Could you check a few things on this model? Use its own coordinates, in mm. A direction names the side the tool comes from. Coordinates: 2 decimals unless noted, no trailing zeros. Loops run counter-clockwise (first coordinate to the right, second up) from the corner with the lowest first, then second, coordinate; pieces in that order, holes last. Notation, with made-up numbers: (-15.5, -10.75) - (2.5, -10.75) arc R28 cw to (2.5, 23.25) - close; hole circle Ø2 at (10.5, 86.5). An arc over 180 degrees is marked (long way). Put each result on its own line as item: value. Start each with the question number.
```python
from build123d import *

# Parameters (mm, degrees)
SKETCH1_W           = 30
SKETCH1_H           = 30
SKETCH1_W_2         = 20
SKETCH1_H_2         = 20
BOSS_EXTRUDE1_DEPTH = 20
BOSS_EXTRUDE2_START = 20
SKETCH1_2_W         = 30
SKETCH1_2_H         = 30
SKETCH1_2_W_2       = 20
SKETCH1_2_H_2       = 20
BOSS_EXTRUDE2_DEPTH = 10
SKETCH3_R           = 2.5
CUT_EXTRUDE1_DEPTH  = 46
SKETCH3_3_R         = 4
SKETCH3_3_R_2       = 2.5
CUT_EXTRUDE2_DEPTH  = 3
CUT_EXTRUDE3_START  = -27
SKETCH3_4_R         = 4
SKETCH3_4_R_2       = 2.5
CUT_EXTRUDE3_DEPTH  = 3
SKETCH4_W           = 10
SKETCH4_H           = 30
BOSS_EXTRUDE3_DEPTH = 50
SKETCH5_R           = 2.5
CUT_EXTRUDE4_DEPTH  = 84.815273071
LPATTERN1_COUNT     = 6
LPATTERN1_PITCH     = 7.5
FILLET1_R           = 15


with BuildPart() as part:
    # Sketch1 → Boss-Extrude1 (new body)
    with BuildSketch(Plane(origin=(0, 0, 0), x_dir=(1, 0, 0), z_dir=(0, 1, 0))):
        Rectangle(SKETCH1_W, SKETCH1_H)
        Rectangle(SKETCH1_W_2, SKETCH1_H_2, mode=Mode.SUBTRACT)
    extrude(amount=BOSS_EXTRUDE1_DEPTH)

    # Sketch1<2> → Boss-Extrude2 (add)
    # profile 1 of 2: a face of its own
    with BuildSketch(Plane(origin=(0, 0, 0), x_dir=(1, 0, 0), z_dir=(0, 1, 0)).offset(BOSS_EXTRUDE2_START)):
        Rectangle(SKETCH1_2_W, SKETCH1_2_H)
        Rectangle(SKETCH1_2_W_2, SKETCH1_2_H_2, mode=Mode.SUBTRACT)
    # profile 2 of 2: a face of its own
    with BuildSketch(Plane(origin=(0, 0, 0), x_dir=(1, 0, 0), z_dir=(0, 1, 0)).offset(BOSS_EXTRUDE2_START)):
        Rectangle(SKETCH1_2_W_2, SKETCH1_2_H_2)
    extrude(amount=BOSS_EXTRUDE2_DEPTH)

    # Sketch3 → Cut-Extrude1 (cut, through all)
    with BuildSketch(Plane(origin=(15, 0, 0), x_dir=(0, 0, -1), z_dir=(1, 0, 0))):
        with Locations((0, 15)):
            Circle(SKETCH3_R)
    extrude(amount=-CUT_EXTRUDE1_DEPTH, mode=Mode.SUBTRACT)

    # Sketch3<3> → Cut-Extrude2 (cut)
    # profile 1 of 2: a face of its own
    with BuildSketch(Plane(origin=(15, 0, 0), x_dir=(0, 0, -1), z_dir=(1, 0, 0))):
        Polygon((-5, 17.886751346), (-5, 12.113248654), (0, 9.226497308), (5, 12.113248654), (5, 17.886751346), (0, 20.773502692), align=None)
        with Locations((0, 15)):
            Circle(SKETCH3_3_R, mode=Mode.SUBTRACT)
    # profile 2 of 2: a face of its own
    with BuildSketch(Plane(origin=(15, 0, 0), x_dir=(0, 0, -1), z_dir=(1, 0, 0))):
        with Locations((0, 15)):
            Circle(SKETCH3_3_R)
        with Locations((0, 15)):
            Circle(SKETCH3_3_R_2, mode=Mode.SUBTRACT)
    extrude(amount=-CUT_EXTRUDE2_DEPTH, mode=Mode.SUBTRACT)

    # Sketch3<4> → Cut-Extrude3 (cut)
    with BuildSketch(Plane(origin=(15, 0, 0), x_dir=(0, 0, -1), z_dir=(1, 0, 0)).offset(CUT_EXTRUDE3_START)):
        with Locations((0, 15)):
            Circle(SKETCH3_4_R)
        with Locations((0, 15)):
            Circle(SKETCH3_4_R_2, mode=Mode.SUBTRACT)
    extrude(amount=-CUT_EXTRUDE3_DEPTH, mode=Mode.SUBTRACT)

    # Sketch4 → Boss-Extrude3 (add)
    with BuildSketch(Plane(origin=(0, 30, 0), x_dir=(1, 0, 0), z_dir=(0, 1, 0))):
        Rectangle(SKETCH4_W, SKETCH4_H)
    extrude(amount=BOSS_EXTRUDE3_DEPTH)

    # Sketch5 → Cut-Extrude4 (cut, through all)
    with BuildSketch(Plane(origin=(5, 0, 0), x_dir=(0, 0, -1), z_dir=(1, 0, 0))):
        with Locations((0, 37.407153601)):
            Circle(SKETCH5_R)
    cut_extrude4 = extrude(amount=-CUT_EXTRUDE4_DEPTH, mode=Mode.SUBTRACT)

    # LPattern1: Cut-Extrude4 ×6
    with Locations(*[(0, i * LPATTERN1_PITCH, 0) for i in range(1, LPATTERN1_COUNT)]):
        add(cut_extrude4, mode=Mode.SUBTRACT)

    # Fillet1
    fillet1_edges = [part.edges().sort_by_distance(p)[0] for p in [
        (0, 80, -15),
        (0, 80, 15),
    ]]
    fillet(fillet1_edges, radius=FILLET1_R - 0.0001)  # a hair under: the kernel refuses the full size


solid = part.part
```
(1) For pin 1 Ø5 at (y, z) = (48.5, -6.5) entering from +X; pin 2 Ø2 at (x, z) = (-9.5, -1.5) entering from +Y; pin 3 Ø12 at (x, z) = (3, -10) entering from +Y, each with a flat end and sliding along its axis, tell me the tip position at first contact or that it passes through.
(2) I want a section at B-B on x = 13. List the corners of the cut face in (y, z) for me, and give its area (3 significant figures).
(3) I want a section at D-D on y = 59. List the corners of the cut face in (x, z) for me.
(4) I want a section at A-A on y = 15. List the corners of the cut face in (x, z) for me.
(5) I need wall thicknesses on L1, parallel to X at y = 16, z = -4; L2, parallel to Y at x = -12.85, z = 0; L3, parallel to X at y = 40, z = -10. Which ranges of each line are inside material? Lowest first, please. Write a range as [from, to].
(6) Which directions (+Z, -Z, +X, -X, +Y, -Y) give clear straight access to the entire face, cutting with the end or side of a thin tool? Please do faces 1 (the flat face through (10, 30, 0)), 2 (the flat face through (-5, 55, 4)), 3 (the cylindrical face through (-13.479, 18.966, 0.521)), 4 (the flat face through (13.521, 10.65, -2.465)).
(7) If we mould it in two halves opening along Z, with no side actions, what happens to faces 5 (the cylindrical face through (0.07, 75.49, 10.72)), 6 (the cylindrical face through (0.07, 75.49, -10.72)), 7 (the flat face through (10, 10, 0))? For each: pulls with the +Z half, pulls with the -Z half, needs draft (parallel to the pull), parting line crosses it, or undercut.
(8) I want a section at C-C on x = 7.5. List the corners of the cut face in (y, z) for me, and give its area (3 significant figures).
Answer sheet:
1. pin 1: stops at x = 5
1. pin 2: stops at y = 30
1. pin 3: stops at y = 79.46
2. outline: (0, -15) - (30, -15) - (30, 15) - (0, 15) - close; hole (9.23, 0) - (12.11, -5) - (17.89, -5) - (20.77, 0) - (17.89, 5) - (12.11, 5) - close
2. area: 813 mm^2
3. outline: (-5, -15) - (5, -15) - (5, -2.33) - (-5, -2.33) - close; (-5, 2.33) - (5, 2.33) - (5, 15) - (-5, 15) - close
4. outline: (-15, -15) - (15, -15) - (15, -5) - (12, -5) - (12, -2.5) - (10, -2.5) - (10, -10) - (-10, -10) - (-10, -2.5) - (-12, -2.5) - (-12, -4) - (-15, -4) - close; (-15, 4) - (-12, 4) - (-12, 2.5) - (-10, 2.5) - (-10, 10) - (10, 10) - (10, 2.5) - (12, 2.5) - (12, 5) - (15, 5) - (15, 15) - (-15, 15) - close
5. L1: x = [-15, -10], [10, 12]
5. L2: y = [0, 11], [19, 30]
5. L3: x = [-5, 5]
6. face 1: +Z, -Z, +X, +Y
6. face 2: +Z, -Z, -X, +Y
6. face 3: -X
6. face 4: +X
7. face 5: pulls with the +Z half
7. face 6: pulls with the -Z half
7. face 7: undercut
8. outline: (0, -15) - (30, -15) - (30, 15) - (0, 15) - (0, 10) - (20, 10) - (20, -10) - (0, -10) - close
8. area: 500 mm^2
